Check sheet for the modelled part. Datum: model origin and axes. Units: mm. A direction names the side the tool comes from. Coordinates: 2 decimals unless noted, no trailing zeros. Loops run counter-clockwise (first coordinate to the right, second up) from the corner with the lowest first, then second, coordinate; pieces in that order, holes last.
```python
from build123d import *

# Parameters (mm, degrees)
SKETCH_1_W          = 5
SKETCH_1_H          = 11.498155491
EXTRUDE_1_DEPTH     = 3.5
SKETCH_2_W          = 1.1
SKETCH_2_H          = 2
CUT_EXTRUDE_1_DEPTH = 4.5
FILLET_1_R          = 0.6
FILLET_2_R          = 0.2


with BuildPart() as part:
    # Sketch 1 → Extrude 1 (new body, symmetric)
    with BuildSketch(Plane.XY):
        with Locations((0, 5.749077746)):
            Rectangle(SKETCH_1_W, SKETCH_1_H)
        with BuildLine():
            Line((-6.75, 0), (-7.5, 1.299038106))
            ThreePointArc((-7.5, 1.299038106), (0, 3.498155491), (7.5, 1.299038106))
            Line((7.5, 1.299038106), (6.75, 0))
            ThreePointArc((6.75, 0), (0, 2), (-6.75, 0))
        make_face()
    extrude(amount=EXTRUDE_1_DEPTH, both=True)

    # Sketch 2 → Cut-Extrude 1 (cut)
    with BuildSketch(Plane.XZ):
        Rectangle(SKETCH_2_W, SKETCH_2_H)
    extrude(amount=-CUT_EXTRUDE_1_DEPTH, mode=Mode.SUBTRACT)

    # Fillet 1
    fillet_1_edges = [part.edges().sort_by_distance(p)[0] for p in [
        (-5.096317816, 2.529350551, 3.5),
        (0, 11.498155491, -3.5),
        (2.5, 7.384728273, -3.5),
        (5.096317816, 2.529350551, -3.5),
        (-7.125, 0.649519053, 3.5),
        (7.125, 0.649519053, -3.5),
        (4.706594524, 1.071292635, -3.5),
        (2.5, 0.872586393, -3.5),
        (0, 0, -3.5),
        (-2.5, 0.872586393, -3.5),
        (-4.706594524, 1.071292635, -3.5),
        (-7.125, 0.649519053, -3.5),
        (-5.096317816, 2.529350551, -3.5),
        (-2.5, 7.384728273, -3.5),
        (-4.706594524, 1.071292635, 3.5),
        (-2.5, 11.498155491, 0),
        (2.5, 11.498155491, 0),
        (2.5, 3.271301055, 0),
        (7.5, 1.299038106, 0),
        (6.75, 0, 0),
        (2.5, 1.745172786, 0),
        (2.5, 0, 0),
        (-2.5, 0, 0),
        (-2.5, 1.745172786, 0),
        (-6.75, 0, 0),
        (-7.5, 1.299038106, 0),
        (-2.5, 3.271301055, 0),
        (-2.5, 0.872586393, 3.5),
        (0, 0, 3.5),
        (2.5, 0.872586393, 3.5),
        (4.706594524, 1.071292635, 3.5),
        (7.125, 0.649519053, 3.5),
        (-2.5, 7.384728273, 3.5),
        (5.096317816, 2.529350551, 3.5),
        (2.5, 7.384728273, 3.5),
        (0, 11.498155491, 3.5),
    ]]
    fillet(fillet_1_edges, radius=FILLET_1_R)

    # Fillet 2
    fillet_2_edges = [part.edges().sort_by_distance(p)[0] for p in [
        (0.55, 0, 0),
        (0, 0, 1),
        (-0.55, 0, 0),
        (0, 0, -1),
    ]]
    fillet(fillet_2_edges, radius=FILLET_2_R)


solid = part.part
```
1) Section check D-D on z = 3.25. Enter the section's corners in (x, y), plus the area to 3 significant figures.
Answer sheet:
outline: (-7.11, 0.85) - (-6.96, 0.59) arc R0.49 ccw to (-6.29, 0.41) arc R12.5 cw to (-3.29, 1.67) arc R0.71 cw to (-2.39, 0.99) - (-2.39, 0.6) arc R0.49 ccw to (-1.9, 0.11) - (1.9, 0.11) arc R0.49 ccw to (2.39, 0.6) - (2.39, 0.99) arc R0.71 cw to (3.29, 1.67) arc R12.5 cw to (6.29, 0.41) arc R0.49 ccw to (6.96, 0.59) - (7.11, 0.85) arc R0.49 ccw to (6.93, 1.51) arc R13.78 ccw to (2.95, 3.07) arc R0.71 cw to (2.39, 3.76) - (2.39, 10.9) arc R0.49 ccw to (1.9, 11.39) - (-1.9, 11.39) arc R0.49 ccw to (-2.39, 10.9) - (-2.39, 3.76) arc R0.71 cw to (-2.95, 3.07) arc R13.78 ccw to (-6.93, 1.51) arc R0.49 ccw to start
area: 66.7 mm2
2) Mould release check, pull along Z, two halves, no side actions. Record for faces 1 (the cylindrical face through (5.014, 2.562, 0.041)), 2 (the flat face through (0, 6, 3.5)), 3 (the flat face through (0, 2, 1)): +Z half, -Z half, draft (parallel to the pull), parting line (faces both ways), or undercut.
Answer sheet:
face 1: draft
face 2: +Z half
face 3: undercut
3) Scan lines: line 1 (Z direction, x = 0.5, y = 0.75); line 2 (X direction, y = 6.5, z = 2.25); line 3 (Y direction, x = -5.75, z = -2). Record each from-to range of solid material in increasing order.
Answer sheet:
line 1: z = -3.5 to -1, 1 to 3.5
line 2: x = -2.5 to 2.5
line 3: y = 0.59 to 2.25
4) Section check A-A on z = 1.75. Enter the section's corners in (x, y), plus the area to 3 significant figures.
Answer sheet:
outline: (-7.21, 0.79) - (-7.06, 0.53) arc R0.6 ccw to (-6.24, 0.32) arc R12.39 cw to (-3.26, 1.56) arc R0.6 cw to (-2.5, 0.99) - (-2.5, 0.6) arc R0.6 ccw to (-1.9, 0) - (1.9, 0) arc R0.6 ccw to (2.5, 0.6) - (2.5, 0.99) arc R0.6 cw to (3.26, 1.56) arc R12.39 cw to (6.24, 0.32) arc R0.6 ccw to (7.06, 0.53) - (7.21, 0.79) arc R0.6 ccw to (6.99, 1.61) arc R13.89 ccw to (2.97, 3.18) arc R0.6 cw to (2.5, 3.76) - (2.5, 10.9) arc R0.6 ccw to (1.9, 11.5) - (-1.9, 11.5) arc R0.6 ccw to (-2.5, 10.9) - (-2.5, 3.76) arc R0.6 cw to (-2.97, 3.18) arc R13.89 ccw to (-6.99, 1.61) arc R0.6 ccw to start
area: 72.3 mm2
5) Section check B-B on y = 6.5. Enter the section's corners in (x, z), plus the area to 3 significant figures.
Answer sheet:
outline: (-2.5, -2.9) arc R0.6 ccw to (-1.9, -3.5) - (1.9, -3.5) arc R0.6 ccw to (2.5, -2.9) - (2.5, 2.9) arc R0.6 ccw to (1.9, 3.5) - (-1.9, 3.5) arc R0.6 ccw to (-2.5, 2.9) - close
area: 34.7 mm2
6) Depth check by flat-ended pin: pin 1 (1.5 mm diameter, centred on y = 8.5, z = 0, fed in from -X); pin 2 (2 mm diameter, centred on y = 6.5, z = -1.5, fed in from +X); pin 3 (1 mm diameter, centred on x = -6, z = -0.5, fed in from +Y); pin 4 (5 mm diameter, centred on x = 2.5, y = 7.5, fed in from -Z). Enter the tip coordinate at first touch or a pass-through.
Answer sheet:
pin 1: stops at x = -2.5
pin 2: stops at x = 2.5
pin 3: stops at y = 2.36
pin 4: stops at z = -3.5
7) Set-up check for faces 4 (the cylindrical face through (-4.767, 1.046, 0.041)), 5 (the flat face through (0, 2, -1)), 6 (the flat face through (-2.5, 7, 0)): record each of +Z, -Z, +X, -X, +Y, -Y from which the full face is reachable in a straight line by a thin tool's end or side.
Answer sheet:
face 4: +Z, -Z, -Y
face 5: -Y
face 6: +Z, -Z, -X, +Y
